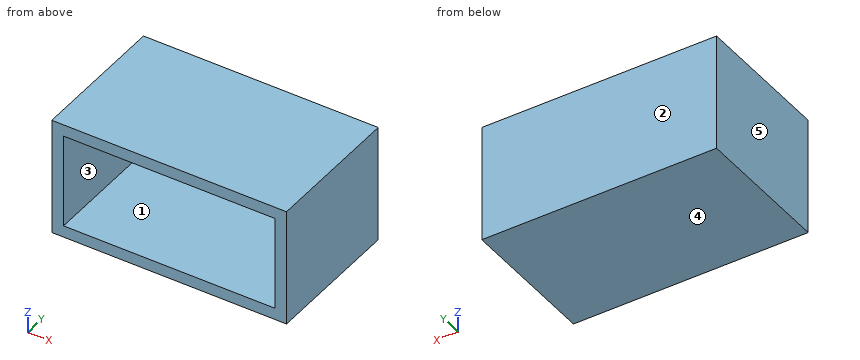
Autodesk Fusion 360 part; units mm, degrees
sketch "スケッチ1" plane through (0, 0, 0) normal (0, 0, 1) x (1, 0, 0)
  line L0 (0, 0) -> (-200, 0)
  line L1 (-200, 0) -> (-200, 120)
  line L2 (-200, 120) -> (0, 120)
  line L3 (0, 120) -> (0, 0)
  dimension "d1" = 200
  dimension "d2" = 120
extrude "押し出し1" add sketch "スケッチ1" along normal blind 10
sketch "スケッチ2" plane through (0, 0, 10) normal (0, 0, 1) x (-1, 0, 0)
  line L0 (0, -120) -> (200, -120)
  line L1 (200, -120) -> (200, 0)
  line L2 (200, 0) -> (0, 0)
  line L3 (0, 0) -> (0, -120)
  line L4 (190, 0) -> (190, -110)
  line L5 (190, -110) -> (10, -110)
  line L6 (10, -110) -> (10, 0)
extrude "押し出し2" add sketch "スケッチ2" along normal blind 90 contours L0 L1 L2 L3 L4 L5 L6
sketch "スケッチ3" plane through (0, 110, 0) normal (0, -1, 0) x (1, 0, 0)
  line L0 (-190, 10) -> (-10, 10)
  line L1 (-10, 10) -> (-10, 100)
  line L2 (-10, 100) -> (-190, 100)
  line L3 (-190, 100) -> (-190, 10)
  line L4 (-190, 90) -> (-10, 90)
  line L5 (-10, 90) -> (-10, 100)
  line L6 (-10, 100) -> (-190, 100)
  line L7 (-190, 100) -> (-190, 90)
extrude "押し出し3" add sketch "スケッチ3" along normal blind 110 contours L1 L2 L3 L4 L5 L6 L7
Check sheet for the modelled part. Datum: model origin and axes. Units: mm. Face numbers are marked on the shaded views. A direction names the side the tool comes from. Give positions to 0.01 mm unless a question says otherwise; leave off trailing zeros. Write each loop counter-clockwise with the first axis right and the second up, starting at its lowest first coordinate (ties: lowest second). Pieces come first, ordered by that corner, then holes. Notation, with made-up numbers: (-17.5, 0.25) -> (32.5, 0.25) arc R9 ccw to (32.5, 14.25) -> close; hole circle Ø1 at (86.25, 11). An arc over 180 degrees is marked (long way). Use one line per item in the form item = value. Start each with the question number.
1. Go/stop test with a flat-tipped pin: P1, Ø24, axis at y = 41, z = 45, coming from the +X side. Record where the tip stops, or that it passes through.
2. Thickness scan on line 1 along Z through (x, y) = (-71, 97.5); line 2 along X through (y, z) = (7, 57); line 3 along Y through (x, z) = (-117, 39). Record the ranges inside material, lowest first. Write a range as from..to.
3. Section check A-A (y = 96). Record the cut outline in (x, z).
4. Section check C-C (z = 82). Record the cut outline in (x, y), and give its area (3 significant figures).
5. Access from +Z, -Z, +X, -X, +Y, -Y to the whole of each face (thin tool, end or side, straight path). Record for the marked faces 1 and 2.
6. Section check B-B (x = -91). Record the cut outline in (y, z).
7. Mould release check, pull along X, two halves, no side actions. Record for the marked faces 3, 4 and 5: pulls with the +X half, pulls with the -X half, needs draft (parallel to the pull), parting line crosses it, or undercut.
Conclusion:
q1.P1 = 0
q2.line_1 = 0..10, 90..100
q2.line_2 = -200..-190, -10..0
q2.line_3 = 110..120
q3.outline = (-200, 0) -> (0, 0) -> (0, 100) -> (-200, 100) -> close; hole (-190, 10) -> (-10, 10) -> (-10, 90) -> (-190, 90) -> close
q4.outline = (-200, 0) -> (-190, 0) -> (-190, 110) -> (-10, 110) -> (-10, 0) -> (0, 0) -> (0, 120) -> (-200, 120) -> close
q4.area = 4,200 mm²
q5.face_1 = -Y
q5.face_2 = +Z, -Z, +X, -X, +Y
q6.outline = (0, 0) -> (120, 0) -> (120, 100) -> (0, 100) -> (0, 90) -> (110, 90) -> (110, 10) -> (0, 10) -> close
q7.face_3 = undercut
q7.face_4 = needs draft
q7.face_5 = pulls with the -X half
